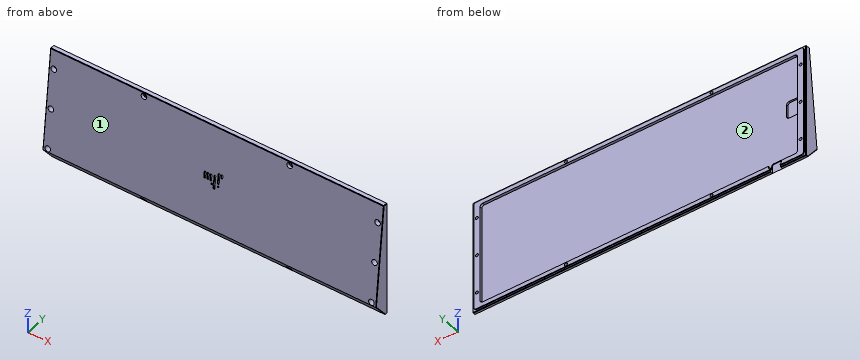
```python
from build123d import *
from OCP.BRepFilletAPI import BRepFilletAPI_MakeChamfer

# Parameters (mm, degrees)
SKETCH1_W            = 390.7
SKETCH1_H            = 132.7
MAINBODY_DEPTH       = 18.5
SKETCH2_W            = 390.7
SKETCH2_H            = 132.7
SKETCH2_W_2          = 386.7
SKETCH2_H_2          = 128.7
ALIGMENTLIP_DEPTH    = 1
TYPINGANGLE_DEPTH    = 414.035143783
SKETCH4_W            = 372
SKETCH4_H            = 119.1
PCBCUTOUT_DEPTH      = 3
M3_CLEARANCE_HOLE1_D = 3.4
CUT_EXTRUDE2_START   = -1
SKETCH11_R           = 3.25
CUT_EXTRUDE2_DEPTH   = 412.911649145
SKETCH13_W           = 15
SKETCH13_H           = 20
CUT_EXTRUDE4_DEPTH   = 2
FILLET2_R            = 3
CHAMFER1_SIZE        = 0.5
CHAMFER1_SIZE2       = 0.561801899
CHAMFER2_SIZE        = 0.1
SKETCH17_R           = 1
SKETCH17_W           = 2
SKETCH17_H           = 2
CUT_EXTRUDE5_DEPTH   = 1
SKETCH18_W           = 12
SKETCH18_H           = 4
CUT_EXTRUDE6_DEPTH   = 10
SKETCH12_W           = 15
SKETCH12_H           = 3.95
CUT_EXTRUDE3_DEPTH   = 3
FILLET1_R            = 2.5


with BuildPart() as part:
    # Sketch1 → MainBody (new body)
    with BuildSketch(Plane(origin=(0, 0, 0), x_dir=(1, 0, 0), z_dir=(0, 1, 0))):
        with Locations((195.35, 66.35)):
            Rectangle(SKETCH1_W, SKETCH1_H)
    extrude(amount=MAINBODY_DEPTH)

    # Sketch2 → AligmentLip (cut)
    with BuildSketch(Plane(origin=(0, 18.5, 0), x_dir=(1, 0, 0), z_dir=(0, 1, 0))):
        with Locations((195.35, 66.35)):
            Rectangle(SKETCH2_W, SKETCH2_H)
        with Locations((195.35, 66.35)):
            Rectangle(SKETCH2_W_2, SKETCH2_H_2, mode=Mode.SUBTRACT)
    extrude(amount=-ALIGMENTLIP_DEPTH, mode=Mode.SUBTRACT)

    # Sketch3 → TypingAngle (cut, through all)
    with BuildSketch(Plane.ZY):
        Polygon((-114.79399123, 0), (-132.7, 14.5), (-132.7, 0), align=None)
        Polygon((0, 12.065334661), (-114.79399123, 0), (0, 0), align=None)
    extrude(amount=-TYPINGANGLE_DEPTH, mode=Mode.SUBTRACT)

    # Sketch4 → PCBCutout (cut)
    with BuildSketch(Plane(origin=(0, 18.5, 0), x_dir=(1, 0, 0), z_dir=(0, 1, 0))):
        with Locations((195.35, 66.35)):
            Rectangle(SKETCH4_W, SKETCH4_H)
    extrude(amount=-PCBCUTOUT_DEPTH, mode=Mode.SUBTRACT)

    # M3 Clearance Hole1 (through all)
    with Locations(Plane(origin=(110, 18.5, -128.3), x_dir=(0, 0, 1), z_dir=(0, 1, 0))):
        with Locations((0, 0), (16.95, -104.3), (61.95, -104.3), (106.95, -104.3), (123.9, 0), (0, 170.7), (123.9, 170.7), (106.95, 275), (61.95, 275), (16.95, 275)):
            Hole(M3_CLEARANCE_HOLE1_D / 2)

    # Sketch11 → Cut-Extrude2 (cut, through all)
    with BuildSketch(Plane(origin=(0, 15.5, 0), x_dir=(1, 0, 0), z_dir=(0, 1, 0)).offset(CUT_EXTRUDE2_START)):
        with Locations(Location((110, 128.3, 0), (0, 0, 270))):
            Circle(SKETCH11_R)
        with Locations(Location((5.7, 111.35, 0), (0, 0, 270))):
            Circle(SKETCH11_R)
        with Locations(Location((5.7, 66.35, 0), (0, 0, 270))):
            Circle(SKETCH11_R)
        with Locations(Location((5.7, 21.35, 0), (0, 0, 270))):
            Circle(SKETCH11_R)
        with Locations(Location((110, 4.4, 0), (0, 0, 270))):
            Circle(SKETCH11_R)
        with Locations(Location((280.7, 4.4, 0), (0, 0, 270))):
            Circle(SKETCH11_R)
        with Locations(Location((385, 21.35, 0), (0, 0, 270))):
            Circle(SKETCH11_R)
        with Locations(Location((385, 66.35, 0), (0, 0, 270))):
            Circle(SKETCH11_R)
        with Locations(Location((385, 111.35, 0), (0, 0, 270))):
            Circle(SKETCH11_R)
        with Locations(Location((280.7, 128.3, 0), (0, 0, 90))):
            Circle(SKETCH11_R)
    extrude(amount=-CUT_EXTRUDE2_DEPTH, mode=Mode.SUBTRACT)

    # Sketch13 → Cut-Extrude4 (cut)
    with BuildSketch(Plane(origin=(0, 15.5, 0), x_dir=(1, 0, 0), z_dir=(0, 1, 0))):
        with Locations((16.85, 66.35)):
            Rectangle(SKETCH13_W, SKETCH13_H)
    extrude(amount=-CUT_EXTRUDE4_DEPTH, mode=Mode.SUBTRACT)

    # Fillet2
    fillet2_edges = [part.edges().sort_by_distance(p)[0] for p in [
        (388.7, 18, -130.7),
        (2, 18, -130.7),
        (2, 18, -2),
        (9.35, 14.5, -56.35),
        (9.35, 14.5, -76.35),
        (24.35, 14.5, -76.35),
        (24.35, 14.5, -56.35),
        (388.7, 18, -2),
        (9.35, 17, -6.8),
        (9.35, 17, -125.9),
        (381.35, 17, -125.9),
        (381.35, 17, -6.8),
    ]]
    fillet(fillet2_edges, radius=FILLET2_R)

    # Chamfer1: one chamfer whose edges measure the first distance from different faces: ONE call of the kernel's chamfer builder (chamfer() names one face for all edges)
    chamfer1_edges_1 = [part.edges().sort_by_distance(p)[0] for p in [
        (0, 16, -132.7),
        (390.7, 16, -132.7),
        (390.7, 14.782667331, 0),
        (0, 14.782667331, 0),
        (195.35, 17.5, -132.7),
        (390.7, 17.5, -66.35),
        (195.35, 17.5, 0),
        (0, 17.5, -66.35),
        (0, 7.25, -123.746995615),
        (390.7, 7.25, -123.746995615),
        (0, 6.032667331, -57.396995615),
        (390.7, 6.032667331, -57.396995615),
    ]]
    chamfer1_edges_2 = [part.edges().sort_by_distance(p)[0] for p in [
        (195.35, 12.065334661, 0),
    ]]
    chamfer1_side_2 = [part.faces().sort_by_distance(p)[0] for p in [
        (195.35, 14.782667331, 0),
    ]]
    chamfer1 = BRepFilletAPI_MakeChamfer(part.part.solid().wrapped)
    for e in chamfer1_edges_1:
        chamfer1.Add(CHAMFER1_SIZE, e.wrapped)
    for e in chamfer1_edges_2:
        chamfer1.Add(CHAMFER1_SIZE, CHAMFER1_SIZE2, e.wrapped, chamfer1_side_2[0].wrapped)  # the first distance lies on this face
    add(Compound.cast(chamfer1.Shape()), mode=Mode.REPLACE)

    # Chamfer2
    chamfer2_edges = [part.edges().sort_by_distance(p)[0] for p in [
        (388.7, 18.5, -66.35),
        (195.35, 18.5, -130.7),
        (2, 18.5, -66.35),
        (195.35, 18.5, -2),
        (2.878679656, 18.5, -129.821320344),
        (2.878679656, 18.5, -2.878679656),
        (387.821320344, 18.5, -2.878679656),
        (387.821320344, 18.5, -129.821320344),
    ]]
    chamfer(chamfer2_edges, length=CHAMFER2_SIZE)

    # Sketch17 → Cut-Extrude5 (cut)
    with BuildSketch(Plane(origin=(0, 11.933506406, -1.254262065), x_dir=(1, 0, 0), z_dir=(0, -0.9945218953682734, 0.10452846326765429))):
        with Locations((205.1, -52.238829109)):
            Circle(SKETCH17_R)
        with BuildLine():
            ThreePointArc((204.1, -52.238829109), (205.1, -51.238829109), (206.1, -52.238829109))
            Line((206.1, -52.238829109), (206.1, -49.738829109))
            ThreePointArc((206.1, -49.738829109), (205.1, -50.738829109), (204.1, -49.738829109))
            Line((204.1, -49.738829109), (204.1, -52.238829109))
        make_face()
        with Locations((205.1, -49.738829109)):
            Circle(SKETCH17_R)
        with Locations((201.6, -49.738829109)):
            Circle(SKETCH17_R)
        with BuildLine():
            ThreePointArc((200.6, -60.238829109), (201.6, -59.238829109), (202.6, -60.238829109))
            Line((202.6, -60.238829109), (202.6, -49.738829109))
            ThreePointArc((202.6, -49.738829109), (201.6, -50.738829109), (200.6, -49.738829109))
            Line((200.6, -49.738829109), (200.6, -60.238829109))
        make_face()
        with Locations((201.6, -60.238829109)):
            Circle(SKETCH17_R)
        with Locations((197.1, -53.738829109)):
            Circle(SKETCH17_R)
        with BuildLine():
            Line((196.1, -62.738829109), (198.1, -62.738829109))
            Line((198.1, -62.738829109), (198.1, -53.738829109))
            ThreePointArc((198.1, -53.738829109), (197.1, -54.738829109), (196.1, -53.738829109))
            Line((196.1, -53.738829109), (196.1, -62.738829109))
        make_face()
        with Locations((197.1, -63.738829109)):
            Rectangle(SKETCH17_W, SKETCH17_H)
        with BuildLine():
            ThreePointArc((196.1, -67.738829109), (197.1, -66.738829109), (198.1, -67.738829109))
            Line((198.1, -67.738829109), (198.1, -64.738829109))
            Line((198.1, -64.738829109), (196.1, -64.738829109))
            Line((196.1, -64.738829109), (196.1, -67.738829109))
        make_face()
        with Locations((197.1, -67.738829109)):
            Circle(SKETCH17_R)
        with BuildLine():
            Line((194.1, -64.738829109), (196.1, -64.738829109))
            Line((196.1, -64.738829109), (196.1, -62.738829109))
            Line((196.1, -62.738829109), (194.1, -62.738829109))
            ThreePointArc((194.1, -62.738829109), (194.807106781, -63.031722328), (195.1, -63.738829109))
            ThreePointArc((195.1, -63.738829109), (194.807106781, -64.44593589), (194.1, -64.738829109))
        make_face()
        with Locations((194.1, -63.738829109)):
            Circle(SKETCH17_R)
        with Locations(Location((201.6, -63.738829109, 0), (0, 0, 270))):
            Circle(SKETCH17_R)
        with Locations((192.6, -60.238829109)):
            Circle(SKETCH17_R)
        with BuildLine():
            ThreePointArc((191.6, -60.238829109), (192.6, -59.238829109), (193.6, -60.238829109))
            Line((193.6, -60.238829109), (193.6, -54.238829109))
            ThreePointArc((193.6, -54.238829109), (192.6, -55.238829109), (191.6, -54.238829109))
            Line((191.6, -54.238829109), (191.6, -60.238829109))
        make_face()
        with Locations((192.6, -54.238829109)):
            Circle(SKETCH17_R)
        with BuildLine():
            ThreePointArc((188.1, -60.238829109), (189.1, -59.238829109), (190.1, -60.238829109))
            Line((190.1, -60.238829109), (190.1, -54.238829109))
            ThreePointArc((190.1, -54.238829109), (189.1, -55.238829109), (188.1, -54.238829109))
            Line((188.1, -54.238829109), (188.1, -60.238829109))
        make_face()
        with Locations((189.1, -60.238829109)):
            Circle(SKETCH17_R)
        with Locations((189.1, -54.238829109)):
            Circle(SKETCH17_R)
        with Locations((185.6, -54.238829109)):
            Circle(SKETCH17_R)
        with BuildLine():
            ThreePointArc((184.6, -60.238829109), (185.6, -59.238829109), (186.6, -60.238829109))
            Line((186.6, -60.238829109), (186.6, -54.238829109))
            ThreePointArc((186.6, -54.238829109), (185.6, -55.238829109), (184.6, -54.238829109))
            Line((184.6, -54.238829109), (184.6, -60.238829109))
        make_face()
        with Locations((185.6, -60.238829109)):
            Circle(SKETCH17_R)
    extrude(amount=-CUT_EXTRUDE5_DEPTH, mode=Mode.SUBTRACT)

    # Sketch18 → Cut-Extrude6 (cut)
    with BuildSketch(Plane(origin=(0, 0, -132.7), x_dir=(-1, 0, 0), z_dir=(0, 0, -1))):
        with Locations((-35.8, 16.5)):
            Rectangle(SKETCH18_W, SKETCH18_H)
    extrude(amount=-CUT_EXTRUDE6_DEPTH, mode=Mode.SUBTRACT)

    # Sketch12 → Cut-Extrude3 (cut)
    with BuildSketch(Plane(origin=(0, 18.5, 0), x_dir=(1, 0, 0), z_dir=(0, 1, 0))):
        with Locations((35.8, 127.875)):
            Rectangle(SKETCH12_W, SKETCH12_H)
    extrude(amount=-CUT_EXTRUDE3_DEPTH, mode=Mode.SUBTRACT)

    # Fillet1
    # the kernel refuses this fillet: 2.5 mm, written as the material it adds along each edge
    with BuildSketch(Plane(origin=(43.3, 18.5, -129.85), x_dir=(-1, 0, 0), z_dir=(0, -1, 0))) as fillet1_piece_1:
        with BuildLine():
            CenterArc((2.5, -2.291287847), FILLET1_R, 113.578178478, 66.421821522)
            Line((0, -2.291287847), (0, 0))
            Line((0, 0), (1.5, 0))
        make_face()
    extrude(amount=3)
    with BuildSketch(Plane(origin=(28.3, 18.5, -129.85), x_dir=(0, 0, 1), z_dir=(0, -1, 0))) as fillet1_piece_2:
        with BuildLine():
            CenterArc((2.291287847, -2.5), FILLET1_R, 90, 66.421821522)
            Line((0, -1.5), (0, 0))
            Line((0, 0), (2.291287847, 0))
        make_face()
    extrude(amount=3)
    with BuildSketch(Plane(origin=(41.8, 14.5, -122.7), x_dir=(-1, 0, 0), z_dir=(0, 1, 0)), Plane(origin=(29.8, 15.5, -122.7), x_dir=(1, 0, 0), z_dir=(0, -1, 0))) as fillet1_piece_3:
        with BuildLine():
            CenterArc((FILLET1_R, -FILLET1_R), FILLET1_R, 90, 90)
            Line((0, -FILLET1_R), (0, 0))
            Line((0, 0), (FILLET1_R, 0))
        make_face()
    extrude(amount=1)


solid = part.part
```
Source: CAD feature listing. Evaluate the final solid. Frame: model axes, mm. Face numbers are marked on the shaded views. Coordinates: 2 decimals unless noted, no trailing zeros. Loops run counter-clockwise (first coordinate to the right, second up) from the corner with the lowest first, then second, coordinate; pieces in that order, holes last. Notation, with made-up numbers: (67.5, -28) -> (95.5, -28) arc R33 cw to (95.5, 11) -> close; hole circle Ø5 at (-19.5, 13.5). An arc over 180 degrees is marked (long way). One line per item, written item: value. Start each with the question number.
Q1. Line query: line 1 along Z through (x, y) = (280.7, 16.65); line 2 along X through (y, z) = (13.5, -4.4); line 3 along X through (y, z) = (15.75, -111). Output: solid intervals per line, ascending.
Q2. Section query B-B, the plane z = -31. Return the cut outline in (x, y).
Q3. Section query A-A, the plane x = 303.5. Return the cut outline in (y, z).
Q4. Mould query, pull axis X, two halves, no side actions, for the marked faces 1 and 2. Classes: pulls with the +X half, pulls with the -X half, needs draft (parallel to the pull), parting line crosses it, or undercut.
Q5. Contact query for flat-ended pins moving along their axis: P1, Ø6, axis at x = 280.7, z = -128.3, coming from the -Y side; P2, Ø5.5, axis at x = 5.7, z = -21.35, coming from the +Y side; P3, Ø6, axis at x = 207.5, z = -57.5, coming from the +Y side; P4, Ø5, axis at x = 281.5, z = -3, coming from the -Y side. Output: stop coordinate, or through.
Results:
1. line 1: -132.7 to -130, -126.6 to -125.9, -6.8 to -6.1, -2.7 to 0
1. line 2: 0 to 106.75, 113.25 to 277.45, 283.95 to 390.7
1. line 3: 0 to 4.04, 7.36 to 9.35, 381.35 to 383.34, 386.66 to 390.7
2. outline: (0, 9.31) -> (0.5, 8.81) -> (390.2, 8.81) -> (390.7, 9.31) -> (390.7, 17) -> (390.2, 17.5) -> (388.7, 17.5) -> (388.7, 18.4) -> (388.6, 18.5) -> (381.35, 18.5) -> (381.35, 15.5) -> (9.35, 15.5) -> (9.35, 18.5) -> (2.1, 18.5) -> (2, 18.4) -> (2, 17.5) -> (0.5, 17.5) -> (0, 17) -> close
3. outline: (0, -114.79) -> (14.5, -132.7) -> (17, -132.7) -> (17.5, -132.2) -> (17.5, -130.7) -> (18.4, -130.7) -> (18.5, -130.6) -> (18.5, -125.9) -> (15.5, -125.9) -> (15.5, -6.8) -> (18.5, -6.8) -> (18.5, -2.1) -> (18.4, -2) -> (17.5, -2) -> (17.5, -0.5) -> (17, 0) -> (12.57, 0) -> (12.01, -0.56) -> close
4. face 1: needs draft
4. face 2: undercut
5. P1: y = 14.5
5. P2: y = 18.5
5. P3: y = 15.5
5. P4: y = 11.67
